Check sheet for the modelled part. Datum: model origin and axes. Units: mm. A direction names the side the tool comes from. Round coordinates to 2 decimals unless told otherwise and drop trailing zeros. Order: outer loops, then holes, each group sorted by start corner. A loop starts at its lowest first (then second) coordinate and runs counter-clockwise, first axis right, second up.
```python
from build123d import *

# Parameters (mm, degrees)
F2_R    = 0.49999
F3_SIZE = 1


# Not quite as in the source:
# - a fillet or chamfer is up to 0.001 mm smaller than in the source, because OpenCascade refuses the exact size


with BuildPart() as f1:
    # F0 (on Top) → F1 (revolve)
    with BuildSketch(Plane.XY):
        Polygon((0, 19.8), (-40, 19.8), (-40, 17.3), (-0.5, 17.3), (-0.5, 16.3), (0, 16.3), (0.5, 16.3), (0.5, 17.3), (40, 17.3), (40, 19.8), align=None)
    revolve(axis=Axis((0, 0, 0), (1, 0, 0)))

    # F2 (radius 0.5 in the source; OpenCascade refuses exactly that, so slightly less here)
    f2_edges = [f1.edges().sort_by_distance(p)[0] for p in [
        (-0.5, -16.3, 0),
        (0.5, -16.3, 0),
    ]]
    fillet(f2_edges, radius=F2_R)

    # F3
    f3_edges = [f1.edges().sort_by_distance(p)[0] for p in [
        (-40, -17.3, 0),
        (40, -17.3, 0),
    ]]
    chamfer(f3_edges, length=F3_SIZE)


solid = f1.part
```
Item 1: Go/stop test with flat-tipped pins: P1, Ø5, axis at x = -22, z = 5.5, coming from the +Y side; P2, Ø1, axis at x = -24.5, z = 15, coming from the -Y side; P3, Ø10, axis at y = -13, z = 6.5, coming from the -X side; P4, Ø5, axis at x = -21.5, y = -12, coming from the -Z side. Record where each tip stops, or that it passes through.
Answer:
P1: stops at y = 19.57
P2: stops at y = -13.48
P3: stops at x = -40
P4: stops at z = -17.37
Item 2: Access from +Z, -Z, +X, -X, +Y, -Y to the whole of each face (thin tool, end or side, straight path). Record for faces 1 (the flat face through (40, -18, -6)), 2 (the cylindrical face through (20, 16.5, 5.2)), 3 (the cylindrical face through (-19.5, 16.5, 5.2)).
Answer:
face 1: +Z, -Z, +X, +Y, -Y
face 2: +X
face 3: -X
Item 3: Sectioned sample at C-C (x = -18.5). Record the cut outline in (y, z).
Answer:
outline: circle Ø39.6 at (0, 0); hole circle Ø34.6 at (0, 0)
Item 4: Release check for a two-part mould opening along Z. For faces 4 (the cylindrical face through (-0.6, 18.9, 5.9)), 5 (the flat face through (-40, 18, -6)), 6 (the flat face through (-0.5, -17, -2)) record: released by +Z, released by -Z, zero draft, split by the parting line, or undercut.
Answer:
face 4: split by the parting line
face 5: zero draft
face 6: undercut
Item 5: Scan lines: line 1 along Z through (x, y) = (-17, 0); line 2 along Z through (x, y) = (0, 0); line 3 along Y through (x, z) = (4.5, 5.5). Record each from-to range of solid material in increasing order.
Answer:
line 1: z = -19.8 to -17.3, 17.3 to 19.8
line 2: z = -19.8 to -16.3, 16.3 to 19.8
line 3: y = -19.02 to -16.4, 16.4 to 19.02
